Could you check a few things on this model? Use its own coordinates, in mm. A direction names the side the tool comes from. Give positions to 0.01 mm unless a question says otherwise; leave off trailing zeros. Write each loop counter-clockwise with the first axis right and the second up, starting at its lowest first coordinate (ties: lowest second). Pieces come first, ordered by that corner, then holes. Notation, with made-up numbers: (10.25, 50) - (59.25, 50) arc R29 cw to (59.25, 72) - close; hole circle Ø11 at (-10.5, -2.5). An arc over 180 degrees is marked (long way). Answer as CSV lines item,"result". Start each with the question number.
Q1. On a 3-axis mill with a long thin cutter (end or side, diameter ignored), from which of +Z, -Z, +X, -X, +Y, -Y can I reach the whole of each face in a straight line? I mean faces 1 (the face through (-3, 3, -30.988)), 2 (the face through (-0.889, 3, -35)), 3 (the face through (0, 6.35, -19)). Say none if no direction works.
Q2. Will these pins go through, and if not, where does the flat tip stop? pin 1 Ø1.9 at (y, z) = (2, -35.5) entering from +X; pin 2 Ø6 at (x, z) = (-11.5, -7.5) entering from -Y; pin 3 Ø1 at (y, z) = (5, -25) entering from -X; pin 4 Ø1 at (x, y) = (10.5, 1.5) entering from -Z.
Q3. Imagine slicing it at D-D on z = -18. List the corners of the cut face in (x, y) for me.
Q4. Imagine slicing it at C-C on z = -30. List the corners of the cut face in (x, y) for me (3 decimals), and give its area (3 significant figures).
Q5. Imagine slicing it at A-A on x = 3. List the corners of the cut face in (y, z) for me, and give its area (3 significant figures).
Q6. Imagine slicing it at B-B on y = 5.5. List the corners of the cut face in (x, z) for me (3 decimals), and give its area (3 significant figures).
Q7. If I drill on line 1 along Z through (x, y) = (-2.5, 5.75); line 2 along X through (y, z) = (1.5, -7.62); line 3 along X through (y, z) = (3.5, -5), over which ranges is the centre line in solid material (lowest first)?
```python
from build123d import *

# Parameters (mm, degrees)
BOSS_EXTRUDE1_DEPTH = 6.35
SKETCH2_R           = 3.0861
CUT_EXTRUDE1_DEPTH  = 7.35
CUT_EXTRUDE2_DEPTH  = 7.35


with BuildPart() as part:
    # Sketch1 → Boss-Extrude1 (new body)
    with BuildSketch(Plane(origin=(0, 0, 0), x_dir=(1, 0, 0), z_dir=(0, 1, 0))):
        with BuildLine():
            Line((-11.850422652, 0), (11.850422652, 0))
            ThreePointArc((11.850422652, 0), (16.714804866, 2.268298678), (18.103951884, 7.452665928))
            Line((18.103951884, 7.452665928), (13.625246574, 32.852665928))
            ThreePointArc((13.625246574, 32.852665928), (11.453418664, 36.614382214), (7.371717342, 38.1))
            Line((7.371717342, 38.1), (-7.371717342, 38.1))
            ThreePointArc((-7.371717342, 38.1), (-11.453418664, 36.614382214), (-13.625246574, 32.852665928))
            Line((-13.625246574, 32.852665928), (-18.103951884, 7.452665928))
            ThreePointArc((-18.103951884, 7.452665928), (-16.714804866, 2.268298678), (-11.850422652, 0))
        make_face()
    extrude(amount=BOSS_EXTRUDE1_DEPTH)

    # Sketch2 → Cut-Extrude1 (cut, through all)
    with BuildSketch(Plane(origin=(0, 6.35, 0), x_dir=(1, 0, 0), z_dir=(0, 1, 0))):
        with Locations((-10.16, 7.62)):
            Circle(SKETCH2_R)
        with Locations((10.16, 7.62)):
            Circle(SKETCH2_R)
    extrude(amount=-CUT_EXTRUDE1_DEPTH, mode=Mode.SUBTRACT)

    # Sketch3 → Cut-Extrude2 (cut, through all)
    with BuildSketch(Plane(origin=(0, 6.35, 0), x_dir=(1, 0, 0), z_dir=(0, 1, 0))):
        Polygon((-0.889, 38.1), (-0.889, 30.988), (-5.715, 30.988), (-5.715, 29.21), (5.715, 29.21), (5.715, 30.988), (0.889, 30.988), (0.889, 38.1), align=None)
    extrude(amount=-CUT_EXTRUDE2_DEPTH, mode=Mode.SUBTRACT)


solid = part.part
```
Conclusion:
1,face 1,"+Y, -Y"
1,face 2,"-Z, +Y, -Y"
1,face 3,"+Z, -Z, +X, -X, +Y"
2,pin 1,"x = 13.07"
2,pin 2,"y = 0"
2,pin 3,"x = -15.1"
2,pin 4,"z = -37.53"
3,outline,"(-16.24, 0) - (16.24, 0) - (16.24, 6.35) - (-16.24, 6.35) - close"
4,outline,"(-14.128, 0) - (-5.715, 0) - (-5.715, 6.35) - (-14.128, 6.35) - close; (5.715, 0) - (14.128, 0) - (14.128, 6.35) - (5.715, 6.35) - close"
4,area,"107 mm^2"
5,outline,"(0, -38.1) - (6.35, -38.1) - (6.35, -30.99) - (0, -30.99) - close; (0, -29.21) - (6.35, -29.21) - (6.35, 0) - (0, 0) - close"
5,area,"231 mm^2"
6,outline,"(-18.104, -7.453) - (-13.625, -32.853) arc R6.35 ccw to (-7.372, -38.1) - (-0.889, -38.1) - (-0.889, -30.988) - (-5.715, -30.988) - (-5.715, -29.21) - (5.715, -29.21) - (5.715, -30.988) - (0.889, -30.988) - (0.889, -38.1) - (7.372, -38.1) arc R6.35 ccw to (13.625, -32.853) - (18.104, -7.453) arc R6.35 ccw to (11.85, 0) - (-11.85, 0) arc R6.35 ccw to start; hole circle Ø6.172 at (-10.16, -7.62); hole circle Ø6.172 at (10.16, -7.62)"
6,area,"1,090 mm^2"
7,line 1,"-38.1 to -30.99, -29.21 to 0"
7,line 2,"-18.07 to -13.25, -7.07 to 7.07, 13.25 to 18.07"
7,line 3,"-18.06 to -11.79, -8.53 to 8.53, 11.79 to 18.06"
